from build123d import *

# Parameters (mm, degrees)
F1_DEPTH = 0.762
F2_R     = 1.905
F4_DEPTH = 2.54
F5_R     = 1.905
F7_DEPTH = 2.54
F8_R     = 1.905


with BuildPart() as f1:
    # F0 (on Top) → F1 (new body)
    with BuildSketch(Plane.XY):
        Polygon((19.05, 32.9955678842), (-19.05, 32.9955678842), (-38.1, 0), (-19.05, -32.9955678842), (19.05, -32.9955678842), (38.1, 0), align=None)
    extrude(amount=F1_DEPTH)

    # F2
    f2_edges = [f1.edges().sort_by_distance(p)[0] for p in [
        (38.1, 0, 0.381),
        (19.05, 32.995568, 0.381),
        (-19.05, 32.995568, 0.381),
        (-38.1, 0, 0.381),
        (-19.05, -32.995568, 0.381),
        (19.05, -32.995568, 0.381),
    ]]
    fillet(f2_edges, radius=F2_R)

    # F3 (on Top) → F4 (join)
    with BuildSketch(Plane.XY):
        Polygon((18.415, 31.8957156214), (-18.415, 31.8957156214), (-36.83, 0), (-18.415, -31.8957156214), (18.415, -31.8957156214), (36.83, 0), align=None)
    extrude(amount=F4_DEPTH)

    # F5
    f5_edges = [f1.edges().sort_by_distance(p)[0] for p in [
        (-18.415, -31.895716, 1.651),
        (18.415, -31.895716, 1.651),
        (36.83, 0, 1.651),
        (-36.83, 0, 1.651),
        (18.415, 31.895716, 1.651),
        (-18.415, 31.895716, 1.651),
    ]]
    fillet(f5_edges, radius=F5_R)


with BuildPart() as f7:
    # F6 (on Top) → F7 (new body)
    with BuildSketch(Plane.XY):
        Polygon((17.907, 31.0158338111), (-17.907, 31.0158338111), (-35.814, 0), (-17.907, -31.0158338111), (17.907, -31.0158338111), (35.814, 0), align=None)
    extrude(amount=F7_DEPTH)

    # F8
    f8_edges = [f7.edges().sort_by_distance(p)[0] for p in [
        (-17.907, -31.015834, 1.27),
        (17.907, -31.015834, 1.27),
        (35.814, 0, 1.27),
        (-35.814, 0, 1.27),
        (17.907, 31.015834, 1.27),
        (-17.907, 31.015834, 1.27),
    ]]
    fillet(f8_edges, radius=F8_R)


with BuildPart() as f7_1:
    # F9: moved
    add(f7.part.moved(Location((0, 0, 0.762))))


with BuildPart() as f1_1:
    add(f1.part)

    # F10: cut F7
    add(f7_1.part, mode=Mode.SUBTRACT)


solid = f1_1.part
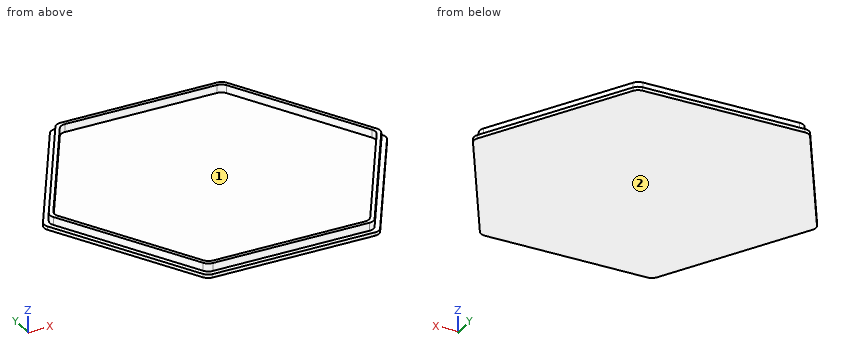
Build history of the part. All positions in model axes, mm. Face numbers are marked on the shaded views. Coordinates: 2 decimals unless noted, no trailing zeros. Write each loop counter-clockwise with the first axis right and the second up, starting at its lowest first coordinate (ties: lowest second). Pieces come first, ordered by that corner, then holes. Notation, with made-up numbers: (-27.5, 47.5) -> (7.5, 47.5) arc R6 ccw to (7.5, 54.5) -> close; hole circle Ø5 at (57.25, 78). An arc over 180 degrees is marked (long way). Use CSV: the item, a comma, the result in double quotes. Start each with the question number.
Q1. Cut at C-C, the plane y = 5. List the corners of the cut face in (x, z).
Q2. Pull direction X, two halves, no side cores. Call the marked faces 1 and 2: released by +X, released by -X, zero draft, split by the parting line, or undercut.
Q3. Flat gauge pins, fed straight in: pin 1 Ø0.9 at (x, z) = (1.5, 2) entering from -Y; pin 2 Ø0.5 at (x, z) = (-0.5, 2) entering from +Y; pin 3 Ø20 at (x, y) = (-14.5, 9.5) entering from +Z. Where does each tip first touch, or does it go through?
Q4. Cut at B-B, the plane x = -8. List the corners of the cut face in (y, z), then the cut area to 3 significant figures.
Q5. Drill centre lines: probe 1 along Y at (x, z) = (16, 1.1); probe 2 along X at (y, z) = (9, 2.15); probe 3 along Z at (x, y) = (17.5, -6). Where is each one in solid material? Low to high.
Q6. Cut at A-A, the plane z = 1.5. List the corners of the cut face in (x, y) (1 decimal).
Checked values:
1,outline,"(-35.21, 0) -> (35.21, 0) -> (35.21, 0.76) -> (33.94, 0.76) -> (33.94, 2.54) -> (32.93, 2.54) -> (32.93, 0.76) -> (-32.93, 0.76) -> (-32.93, 2.54) -> (-33.94, 2.54) -> (-33.94, 0.76) -> (-35.21, 0.76) -> close"
2,face 1,"undercut"
2,face 2,"zero draft"
3,pin 1,"stops at y = -31.9"
3,pin 2,"stops at y = 31.9"
3,pin 3,"stops at z = 0.76"
4,outline,"(-33, 0) -> (33, 0) -> (33, 0.76) -> (31.9, 0.76) -> (31.9, 2.54) -> (31.02, 2.54) -> (31.02, 0.76) -> (-31.02, 0.76) -> (-31.02, 2.54) -> (-31.9, 2.54) -> (-31.9, 0.76) -> (-33, 0.76) -> close"
4,area,"53.4 mm²"
5,probe 1,"y = -31.9 to -31.02, 31.02 to 31.9"
5,probe 2,"x = -31.63 to -30.62, 30.62 to 31.63"
5,probe 3,"z = 0 to 0.76"
6,outline,"(-36.3, -1) -> (-19, -30.9) arc R1.9 ccw to (-17.3, -31.9) -> (17.3, -31.9) arc R1.9 ccw to (19, -30.9) -> (36.3, -1) arc R1.9 ccw to (36.3, 1) -> (19, 30.9) arc R1.9 ccw to (17.3, 31.9) -> (-17.3, 31.9) arc R1.9 ccw to (-19, 30.9) -> (-36.3, 1) arc R1.9 ccw to start; hole (-35.3, -1) -> (-18.5, -30.1) arc R1.9 ccw to (-16.8, -31) -> (16.8, -31) arc R1.9 ccw to (18.5, -30.1) -> (35.3, -1) arc R1.9 ccw to (35.3, 1) -> (18.5, 30.1) arc R1.9 ccw to (16.8, 31) -> (-16.8, 31) arc R1.9 ccw to (-18.5, 30.1) -> (-35.3, 1) arc R1.9 ccw to start"
